Check sheet for the modelled part. Datum: model origin and axes. Units: mm. Coordinates: 2 decimals unless noted, no trailing zeros. Loops run counter-clockwise (first coordinate to the right, second up) from the corner with the lowest first, then second, coordinate; pieces in that order, holes last.
```python
from build123d import *

# Parameters (mm, degrees)
SKETCH1_W                  = 127
SKETCH1_H                  = 762
BOSS_EXTRUDE1_DEPTH        = 25.4
F_1_2_0_5_DIAMETER_HOLE1_D = 50.8
F_1_2_0_5_DIAMETER_HOLE2_D = 12.7


with BuildPart() as part:
    # Sketch1 → Boss-Extrude1 (new body)
    with BuildSketch(Plane(origin=(0, 0, 0), x_dir=(1, 0, 0), z_dir=(0, 1, 0))):
        with Locations((-63.5, 381)):
            Rectangle(SKETCH1_W, SKETCH1_H)
    extrude(amount=BOSS_EXTRUDE1_DEPTH)

    # 1/2 (0.5) Diameter Hole1 (through all)
    with Locations(Plane(origin=(-63.5, 25.4, -698.5), x_dir=(0, 0, 1), z_dir=(0, 1, 0))):
        with Locations((0, 0)):
            Hole(F_1_2_0_5_DIAMETER_HOLE1_D / 2)

    # 1/2 (0.5) Diameter Hole2 (through all)
    with Locations(Plane(origin=(0, 25.4, 0), x_dir=(1, 0, 0), z_dir=(0, 1, 0))):
        with Locations((-103.026104377, 603.131071739), (-64.620447093, 374.288503187), (-26.214789808, 603.131071739), (-26.214789808, 533.157431448), (-103.026104377, 533.157431448), (-64.620447093, 323.488503187), (-64.620447093, 272.688503187), (-64.620447093, 221.888503187), (-64.620447093, 171.088503187), (-64.620447093, 120.288503187), (-64.620447093, 69.488503187), (-64.620447093, 18.688503187), (-64.620447093, -32.111496813)):
            Hole(F_1_2_0_5_DIAMETER_HOLE2_D / 2)


solid = part.part
```
1) Scan lines: line 1 (Z direction, x = -26, y = 20); line 2 (Z direction, x = -108.5, y = 2.25); line 3 (Z direction, x = -86.5, y = 22.25). Record each from-to range of solid material in increasing order.
Answer sheet:
line 1: z = -762 to -609.48, -596.78 to -539.5, -526.81 to 0
line 2: z = -762 to -606.35, -599.91 to -536.38, -529.94 to 0
line 3: z = -762 to -709.28, -687.72 to 0
2) Mould release check, pull along Z, two halves, no side actions. Record for faces 1 (the cylindrical face through (-58.277, 12.522, -18.968)), 2 (the flat face through (0, 13, -376)), 3 (the flat face through (-64, 13, 0)): +Z half, -Z half, draft (parallel to the pull), parting line (faces both ways), or undercut.
Answer sheet:
face 1: undercut
face 2: draft
face 3: +Z half
3) Section check B-B on y = 20.25. Give the number of separate pieces and of enclosed holes in the cut face, plus the area to 3 significant figures.
Answer sheet:
separate pieces: 1
enclosed holes: 13
area: 93,200 mm2
4) Section check A-A on z = -698.5. Enter the section's corners in (x, y), plus the area to 3 significant figures.
Answer sheet:
outline: (-127, 0) - (-88.9, 0) - (-88.9, 25.4) - (-127, 25.4) - close; (-38.1, 0) - (0, 0) - (0, 25.4) - (-38.1, 25.4) - close
area: 1,940 mm2
